```python
from build123d import *

# Parameters (mm, degrees)
SKETCH_1_W            = 30
SKETCH_1_H            = 30
EXTRUDE_1_DEPTH       = 86.25
SKETCH_2_R            = 8.25
CUT_EXTRUDE_1_DEPTH   = 2.5
SKETCH_3_W            = 10
SKETCH_3_H            = 66.25
SKETCH_3_H_2          = 20
CUT_EXTRUDE_2_DEPTH   = 93.542220094
SKETCH_4_W            = 10
SKETCH_4_H            = 20
EXTRUDE_2_DEPTH       = 30
SKETCH_5_W            = 7
SKETCH_5_H            = 86.25
EXTRUDE_3_DEPTH       = 30
SKETCH_6_W            = 27
SKETCH_6_H            = 30
EXTRUDE_4_DEPTH       = 11
SKETCH_7_W            = 20.5
SKETCH_7_H            = 36
CUT_EXTRUDE_3_DEPTH   = 24.7
SKETCH_8_R            = 1.1
SKETCH_8_R_2          = 1.15
CUT_EXTRUDE_4_DEPTH   = 23
SKETCH_9_R            = 8.25
CUT_EXTRUDE_5_DEPTH   = 2.5
SKETCH_10_R           = 1.1
CUT_EXTRUDE_6_DEPTH   = 10
CUT_EXTRUDE_7_DEPTH   = 94.931158302
SKETCH_12_W           = 4.75
SKETCH_12_H           = 91.25
EXTRUDE_5_DEPTH       = 28.7
SKETCH_14_W           = 20.5
SKETCH_14_H           = 5
EXTRUDE_6_DEPTH       = 28.7
CUT_EXTRUDE_9_DEPTH   = 94.931158302
CHAMFER_1_SIZE        = 4
SKETCH_15_R           = 7.5
SKETCH_15_R_2         = 2.5
CUT_EXTRUDE_10_DEPTH  = 93.128999235
SKETCH_16_W           = 9
SKETCH_16_H           = 12.5
CUT_EXTRUDE_11_DEPTH  = 10
CHAMFER_2_SIZE        = 2
SKETCH_18_OUTSIDE_W   = 54.278
SKETCH_18_OUTSIDE_H   = 53.278
SKETCH_18_OUTSIDE_W_2 = 20
SKETCH_18_OUTSIDE_H_2 = 20
CUT_EXTRUDE_12_DEPTH  = 2.5


with BuildPart() as part:
    # 草图1 → 凸台-拉伸1 (new body)
    with BuildSketch(Plane(origin=(0, 0, 0), x_dir=(1, 0, 0), z_dir=(0, 1, 0))):
        Rectangle(SKETCH_1_W, SKETCH_1_H)
    extrude(amount=EXTRUDE_1_DEPTH)

    # 草图2 → 切除-拉伸1 (cut)
    with BuildSketch(Plane(origin=(0, 86.25, 0), x_dir=(1, 0, 0), z_dir=(0, 1, 0))):
        with Locations(Location((1, 0, 0), (0, 0, 270))):
            Circle(SKETCH_2_R)
    extrude(amount=-CUT_EXTRUDE_1_DEPTH, mode=Mode.SUBTRACT)

    # 草图3 → 切除-拉伸2 (cut, through all)
    with BuildSketch(Plane(origin=(0, 0, -15), x_dir=(-1, 0, 0), z_dir=(0, 0, -1))):
        with Locations((10, 33.125)):
            Rectangle(SKETCH_3_W, SKETCH_3_H)
        with Locations((-10, 76.25)):
            Rectangle(SKETCH_3_W, SKETCH_3_H_2)
    extrude(amount=-CUT_EXTRUDE_2_DEPTH, mode=Mode.SUBTRACT)

    # 草图4 → 凸台-拉伸2 (add, through all)
    with BuildSketch(Plane(origin=(0, 0, -15), x_dir=(-1, 0, 0), z_dir=(0, 0, -1))):
        with Locations((-10, 76.25)):
            Rectangle(SKETCH_4_W, SKETCH_4_H)
    extrude(amount=-EXTRUDE_2_DEPTH)

    # 草图5 → 凸台-拉伸3 (add, through all)
    with BuildSketch(Plane(origin=(0, 0, -15), x_dir=(-1, 0, 0), z_dir=(0, 0, -1))):
        with Locations((-18.5, 43.125)):
            Rectangle(SKETCH_5_W, SKETCH_5_H)
    extrude(amount=-EXTRUDE_3_DEPTH)

    # 草图6 → 凸台-拉伸4 (add)
    with BuildSketch(Plane.XZ):
        with Locations((8.5, 0)):
            Rectangle(SKETCH_6_W, SKETCH_6_H)
    extrude(amount=EXTRUDE_4_DEPTH)

    # 草图7 → 切除-拉伸3 (cut)
    with BuildSketch(Plane.ZY.offset(5)):
        with Locations((0, 7)):
            Rectangle(SKETCH_7_W, SKETCH_7_H)
    extrude(amount=-CUT_EXTRUDE_3_DEPTH, mode=Mode.SUBTRACT)

    # 草图8 → 切除-拉伸4 (cut)
    with BuildSketch(Plane.ZY.offset(-19.7)):
        with Locations((-8, -7.5)):
            Circle(SKETCH_8_R)
        with Locations((-8, 22.5)):
            Circle(SKETCH_8_R_2)
        with Locations(Location((8, 22.5, 0), (0, 0, 180))):
            Circle(SKETCH_8_R_2)
        with Locations(Location((8, -7.5, 0), (0, 0, 180))):
            Circle(SKETCH_8_R)
    extrude(amount=-CUT_EXTRUDE_4_DEPTH, mode=Mode.SUBTRACT)

    # 草图9 → 切除-拉伸5 (cut)
    with BuildSketch(Plane(origin=(0, 86.25, 0), x_dir=(1, 0, 0), z_dir=(0, 1, 0))):
        with Locations(Location((1, 0, 0), (0, 0, 270))):
            Circle(SKETCH_9_R)
    extrude(amount=-CUT_EXTRUDE_5_DEPTH, mode=Mode.SUBTRACT)

    # 草图10 → 切除-拉伸6 (cut)
    with BuildSketch(Plane(origin=(0, 83.75, 0), x_dir=(1, 0, 0), z_dir=(0, 1, 0))):
        with Locations(Location((1, 6, 0), (0, 0, 270))):
            Circle(SKETCH_10_R)
        with Locations(Location((7, 0, 0), (0, 0, 270))):
            Circle(SKETCH_10_R)
        with Locations(Location((1, -6, 0), (0, 0, 90))):
            Circle(SKETCH_10_R)
        with Locations(Location((-5, 0, 0), (0, 0, 90))):
            Circle(SKETCH_10_R)
    extrude(amount=-CUT_EXTRUDE_6_DEPTH, mode=Mode.SUBTRACT)

    # 草图11 → 切除-拉伸7 (cut, through all)
    with BuildSketch(Plane(origin=(0, 0, -15), x_dir=(-1, 0, 0), z_dir=(0, 0, -1))):
        Polygon((9, 86.25), (9, 80.25), (-18, 80.25), (-18, -11), (15, -11), (15, 86.25), align=None)
    extrude(amount=-CUT_EXTRUDE_7_DEPTH, mode=Mode.SUBTRACT)

    # 草图12 → 凸台-拉伸5 (add, through all)
    with BuildSketch(Plane.ZY.offset(-19.7)):
        with Locations((-12.625, 34.625)):
            Rectangle(SKETCH_12_W, SKETCH_12_H)
        with Locations((12.625, 34.625)):
            Rectangle(SKETCH_12_W, SKETCH_12_H)
    extrude(amount=EXTRUDE_5_DEPTH)

    # 草图14 → 凸台-拉伸6 (add, through all)
    with BuildSketch(Plane.ZY.offset(-19.7)):
        with Locations((0, 27.5)):
            Rectangle(SKETCH_14_W, SKETCH_14_H)
    extrude(amount=EXTRUDE_6_DEPTH)

    # 草图13 → 切除-拉伸9 (cut, through all)
    with BuildSketch(Plane(origin=(0, 0, -15), x_dir=(-1, 0, 0), z_dir=(0, 0, -1))):
        Polygon((9, 80.25), (-19.7, 15), (-19.7, -11), (9, -11), align=None)
    extrude(amount=-CUT_EXTRUDE_9_DEPTH, mode=Mode.SUBTRACT)

    # 倒角1
    chamfer_1_edges = [part.edges().sort_by_distance(p)[0] for p in [
        (20.85, -11, -15),
        (20.85, -11, 15),
    ]]
    chamfer(chamfer_1_edges, length=CHAMFER_1_SIZE)

    # 草图15 → 切除-拉伸10 (cut, through all)
    with BuildSketch(Plane.ZY.offset(-19.7)):
        with Locations((0, 40.482891964)):
            Circle(SKETCH_15_R)
        with Locations((0, 65.138202804)):
            Circle(SKETCH_15_R_2)
    extrude(amount=-CUT_EXTRUDE_10_DEPTH, mode=Mode.SUBTRACT)

    # 草图16 → 切除-拉伸11 (cut)
    with BuildSketch(Plane.ZY.offset(-19.7)):
        with Locations((10.5, 8.75)):
            Rectangle(SKETCH_16_W, SKETCH_16_H)
        with Locations((-10.5, 8.75)):
            Rectangle(SKETCH_16_W, SKETCH_16_H)
    extrude(amount=-CUT_EXTRUDE_11_DEPTH, mode=Mode.SUBTRACT)

    # 倒角2
    chamfer_2_edges = [part.edges().sort_by_distance(p)[0] for p in [
        (20.85, 2.5, -15),
        (20.85, 2.5, 15),
    ]]
    chamfer(chamfer_2_edges, length=CHAMFER_2_SIZE)

    # 草图18 outside → 切除-拉伸12 (cut)
    with BuildSketch(Plane(origin=(0, 86.25, 0), x_dir=(1, 0, 0), z_dir=(0, 1, 0))):
        with Locations((6.5, 0)):
            Rectangle(SKETCH_18_OUTSIDE_W, SKETCH_18_OUTSIDE_H)
        with Locations((1, 0)):
            Rectangle(SKETCH_18_OUTSIDE_W_2, SKETCH_18_OUTSIDE_H_2, mode=Mode.SUBTRACT)
    extrude(amount=-CUT_EXTRUDE_12_DEPTH, mode=Mode.SUBTRACT)


solid = part.part
```
The model under review builds one solid part; all positions refer to its coordinate system, in mm. A direction names the side the tool comes from. Give positions to 0.01 mm unless a question says otherwise; leave off trailing zeros. Write each loop counter-clockwise with the first axis right and the second up, starting at its lowest first coordinate (ties: lowest second). Pieces come first, ordered by that corner, then holes.
(1) Tool access review of faces 5 (the flat face through (21, 2.5, 9)), 6 (the flat face through (16, 30, 0)), 7 (the flat face through (22, 37, -7)), 8 (the flat face through (19.7, 7, 0)), 9 (the flat face through (21, 2.5, -10)): name each direction out of +Z, -Z, +X, -X, +Y, -Y from which nothing blocks a thin tool from reaching the whole face with its end or side.
(2) Consider section D-D, the plane y = 45. Give the boundary of the cut face in (x, z), and give its area (3 significant figures).
(3) To check wall thickness, follow L1, parallel to Y at x = 21, z = 8; L2, parallel to X at y = 81.65, z = -6; L3, parallel to Z at x = 11, y = 63.5. State the ranges of each line that lie inside material, in increasing order.
(4) The part is to be moulded in two halves that separate along Z. For faces 1 (the flat face through (21, 9, 6)), 2 (the flat face through (21, -11, 0)), 3 (the flat face through (10, 57, -15)), 4 (the cylindrical face through (20.83, 23.52, 7.47)), say which applies: released by +Z, released by -Z, zero draft, split by the parting line, or undercut.
(5) Consider section C-C, the plane y = 22.5. Give the boundary of the cut face in (x, z), and give its area (3 significant figures).
(6) Consider section B-B, the plane x = 7. Give the boundary of the cut face in (y, z), and give its area (3 significant figures).
(7) Consider section A-A, the plane z = 0. Give the number of separate pieces and of enclosed holes in the cut face, and give its area (3 significant figures).
(8) For P1, Ø8, axis at x = 6.5, y = 43.5, coming from the +Z side; P2, Ø8, axis at x = 7, z = 3, coming from the -Y side; P3, Ø5, axis at y = 17.5, z = 5.5, coming from the -X side; P4, Ø2, axis at y = 85.5, z = 1, coming from the +X side, all flat-tipped, find the tip position at first contact; note any pin that passes through.
Returned:
1. face 5: +Z, +X, -X
1. face 6: -X
1. face 7: +Z, -Z, +X, +Y, -Y
1. face 8: -X, -Y
1. face 9: -Z, +X, -X
2. outline: (6.5, -15) - (22, -15) - (22, -5.99) - (19.7, -5.99) - (19.7, 5.99) - (22, 5.99) - (22, 15) - (6.5, 15) - (6.5, 10.25) - (18, 10.25) - (18, -10.25) - (6.5, -10.25) - close
2. area: 202 mm2
3. L1: y = -11 to -8.6, -6.4 to 2.5, 15 to 21.35, 23.65 to 83.75
3. L2: x = -9 to -0.1, 2.1 to 22
3. L3: z = -15 to -10.25, 10.25 to 15
4. face 1: released by +Z
4. face 2: zero draft
4. face 3: released by -Z
4. face 4: undercut
5. outline: (16.4, -15) - (22, -15) - (22, -9.15) - (19.7, -9.15) - (19.7, -10.25) - (16.4, -10.25) - close; (16.4, 10.25) - (19.7, 10.25) - (19.7, 9.15) - (22, 9.15) - (22, 15) - (16.4, 15) - close; (19.7, -6.85) - (22, -6.85) - (22, 6.85) - (19.7, 6.85) - close
5. area: 89.8 mm2
6. outline: (43.87, -15) - (83.75, -15) - (83.75, -10) - (86.25, -10) - (86.25, -5.66) - (83.75, -5.66) - (83.75, -1.1) - (80.25, -1.1) - (80.25, -10.25) - (43.87, -10.25) - close; (43.87, 10.25) - (80.25, 10.25) - (80.25, 1.1) - (83.75, 1.1) - (83.75, 5.66) - (86.25, 5.66) - (86.25, 10) - (83.75, 10) - (83.75, 15) - (43.87, 15) - close
6. area: 465 mm2
7. separate pieces: 3
7. enclosed holes: 0
7. area: 379 mm2
8. P1: stops at z = 15
8. P2: stops at y = 80.25
8. P3: stops at x = 19.7
8. P4: stops at x = 11
